Geometry: final body of the model. Coordinates: model frame, mm. A direction names the side the tool comes from. Give positions to 0.01 mm unless a question says otherwise; leave off trailing zeros. Loops run counter-clockwise (first coordinate to the right, second up) from the corner with the lowest first, then second, coordinate; pieces in that order, holes last.
from build123d import *

# Parameters (mm, degrees)
SKETCH_W        = 78
SKETCH_H        = 48.3
PAD_DEPTH       = 2
SKETCH001_R     = 1.45
POCKET_DEPTH    = 2.001
SKETCH002_R     = 2.85
SKETCH002_R_2   = 1.45
PAD001_DEPTH    = 3
POCKET001_DEPTH = 2.001


with BuildPart() as part:
    # Sketch → Pad (new body)
    with BuildSketch(Plane.XY):
        Rectangle(SKETCH_W, SKETCH_H)
    extrude(amount=PAD_DEPTH)

    # Sketch001 (on Face6 of Pad) → Pocket (cut, through all)
    with BuildSketch(Plane.XY.offset(2)):
        with Locations((-35.57, 20.32)):
            Circle(SKETCH001_R)
        with Locations((35.57, 20.32)):
            Circle(SKETCH001_R)
        with Locations((-35.57, -20.32)):
            Circle(SKETCH001_R)
        with Locations((35.57, -20.32)):
            Circle(SKETCH001_R)
    extrude(amount=-POCKET_DEPTH, mode=Mode.SUBTRACT)

    # Sketch002 (on Face5 of Pocket) → Pad001 (join)
    with BuildSketch(Plane.XY.offset(2)):
        with Locations((-35.57, 20.32)):
            Circle(SKETCH002_R)
        with Locations((-35.57, 20.32)):
            Circle(SKETCH002_R_2, mode=Mode.SUBTRACT)
        with Locations((35.57, 20.32)):
            Circle(SKETCH002_R)
        with Locations((35.57, 20.32)):
            Circle(SKETCH002_R_2, mode=Mode.SUBTRACT)
        with Locations((35.57, -20.32)):
            Circle(SKETCH002_R)
        with Locations((35.57, -20.32)):
            Circle(SKETCH002_R_2, mode=Mode.SUBTRACT)
        with Locations((-35.57, -20.32)):
            Circle(SKETCH002_R)
        with Locations((-35.57, -20.32)):
            Circle(SKETCH002_R_2, mode=Mode.SUBTRACT)
    extrude(amount=PAD001_DEPTH)

    # Sketch003 (on Face5 of Pad001) → Pocket001 (cut, through all)
    with BuildSketch(Plane.XY.offset(2)):
        with BuildLine():
            Line((-27.578066, 20.15), (27.578066, 20.15))
            ThreePointArc((35, 12.728066), (32.826166, 17.976166), (27.578066, 20.15))
            Line((35, 12.728066), (35, -12.728066))
            ThreePointArc((27.578066, -20.15), (32.826166, -17.976166), (35, -12.728066))
            Line((27.578066, -20.15), (-27.578066, -20.15))
            ThreePointArc((-35, -12.728066), (-32.826166, -17.976166), (-27.578066, -20.15))
            Line((-35, -12.728066), (-35, 12.728066))
            ThreePointArc((-27.578066, 20.15), (-32.826166, 17.976166), (-35, 12.728066))
        make_face()
    extrude(amount=-POCKET001_DEPTH, mode=Mode.SUBTRACT)


solid = part.part
Item 1: Section query C-C on x = -23.5. Return loops of the section in (y, z), plus the area to 3 significant figures.
Values follow:
outline: (-24.15, 0) - (-20.15, 0) - (-20.15, 2) - (-24.15, 2) - close; (20.15, 0) - (24.15, 0) - (24.15, 2) - (20.15, 2) - close
area: 16.0 mm2
Item 2: Draft query along Y for faces 4 (the face through (0, 22, 0)), 5 (the face through (-38.417, -20.195, 3.479)), 6 (the face through (-1, 24.15, 1)). Return one class per face: +Y half, -Y half, draft (parallel to the pull), parting line (faces both ways), or undercut.
Values follow:
face 4: draft
face 5: undercut
face 6: +Y half
Item 3: Section query A-A on z = 3.1. Return loops of the section in (x, y), plus the area to 3 significant figures.
Values follow:
outline: circle Ø5.7 at (-35.57, -20.32); circle Ø5.7 at (-35.57, 20.32); circle Ø5.7 at (35.57, -20.32); circle Ø5.7 at (35.57, 20.32); hole circle Ø2.9 at (-35.57, -20.32); hole circle Ø2.9 at (-35.57, 20.32); hole circle Ø2.9 at (35.57, -20.32); hole circle Ø2.9 at (35.57, 20.32)
area: 75.6 mm2
Item 4: Set-up query: faces 1 (the face through (-32.9, -17.9, 1)), 2 (the face through (34, 21, 5)), 3 (the face through (-3, 22, 2)). Return all of +Z, -Z, +X, -X, +Y, -Y with unobstructed straight access to the full face (end or side cutting, diameter ignored); none if empty.
Values follow:
face 1: +Z, -Z
face 2: +Z, +X, -X, +Y, -Y
face 3: +Z
Item 5: Pin query (flat end, axial travel): pin 1 (24 mm diameter, centred on x = 11, y = -11.5, fed in from +Z). Return the tip coordinate at first contact, or that it passes through.
Values follow:
pin 1: stops at z = 2
Item 6: Section query B-B on y = -8.5. Return loops of the section in (x, z).
Values follow:
outline: (-39, 0) - (-35, 0) - (-35, 2) - (-39, 2) - close; (35, 0) - (39, 0) - (39, 2) - (35, 2) - close
Item 7: Ray query, probe 1 along Y at (x, z) = (35.57, 3); probe 2 along X at (y, z) = (4, 1.6); probe 3 along X at (y, z) = (-19.5, 4.1). Return the intervals inside material, ascending.
Values follow:
probe 1: y = -23.17 to -21.77, -18.87 to -17.47, 17.47 to 18.87, 21.77 to 23.17
probe 2: x = -39 to -35, 35 to 39
probe 3: x = -38.3 to -36.77, -34.37 to -32.84, 32.84 to 34.37, 36.77 to 38.3
